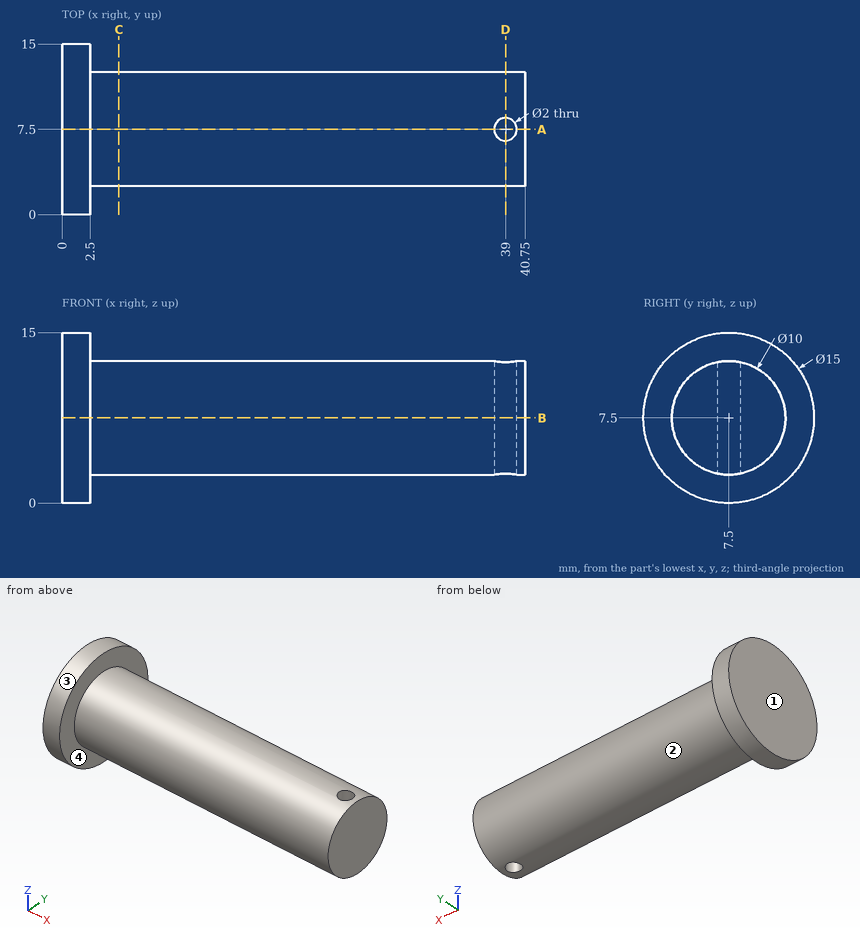
Geometry check sheet. Reference: drawing and pictorial views, mm from the part's lowest x, y, z. A direction names the side the tool comes from. Give positions to 0.01 mm unless a question says otherwise; leave off trailing zeros. Write each loop counter-clockwise with the first axis right and the second up, starting at its lowest first coordinate (ties: lowest second). Pieces come first, ordered by that corner, then holes. Notation, with made-up numbers: (82.5, -35.75) - (99.5, -35.75) arc R15 cw to (99.5, -24.75) - close; hole circle Ø4 at (-0.5, 49.5). An arc over 180 degrees is marked (long way). Put each result on its own line as item: value.
Q1. Section check A-A on y = 7.5. Record the cut outline in (x, z).
Result:
outline: (0, 0) - (2.5, 0) - (2.5, 2.5) - (38, 2.5) - (38, 12.5) - (2.5, 12.5) - (2.5, 15) - (0, 15) - close; (40, 2.5) - (40.75, 2.5) - (40.75, 12.5) - (40, 12.5) - close
Q2. Mould release check, pull along Y, two halves, no side actions. Record for the marked faces 1 and 2: released by +Y, released by -Y, zero draft, split by the parting line, or undercut.
Result:
face 1: zero draft
face 2: split by the parting line
Q3. Set-up check for the marked faces 3 and 4: record each of +Z, -Z, +X, -X, +Y, -Y from which the full face is reachable in a straight line by a thin tool's end or side.
Result:
face 3: +X, -X
face 4: +X
Q4. Section check C-C on x = 5. Record the cut outline in (y, z), and give its area (3 significant figures).
Result:
outline: circle Ø10 at (7.5, 7.5)
area: 78.5 mm2
Q5. Depth check by flat-ended pin: P1, Ø2, axis at x = 30, z = 5.5, coming from the -Y side; P2, Ø2.5, axis at x = 39, y = 7.5, coming from the +Z side; P3, Ø1, axis at x = 24, z = 4, coming from the +Y side. Enter the tip coordinate at first touch or a pass-through.
Result:
P1: y = 2.6
P2: z = 12.5
P3: y = 11.5
Q6. Section check B-B on z = 7.5. Record the cut outline in (x, y).
Result:
outline: (0, 0) - (2.5, 0) - (2.5, 2.5) - (40.75, 2.5) - (40.75, 12.5) - (2.5, 12.5) - (2.5, 15) - (0, 15) - close; hole circle Ø2 at (39, 7.5)
Q7. Section check D-D on x = 39. Record the cut outline in (y, z).
Result:
outline: (6.5, 2.6) - (6.5, 12.4) arc R5 ccw to start; (8.5, 2.6) arc R5 ccw to (8.5, 12.4) - close
Q8. Scan lines: probe 1 along X at (y, z) = (7.5, 6); probe 2 along X at (y, z) = (3.25, 4.75); probe 3 along Y at (x, z) = (39, 5.5). Record each from-to range of solid material in increasing order. Write a range as from..to.
Result:
probe 1: 0..38, 40..40.75
probe 2: 0..2.5
probe 3: 2.92..6.5, 8.5..12.08
